The listing builds one solid part. Answer for the finished solid, in the listing's coordinates (mm). A direction names the side the tool comes from. Coordinates: 2 decimals unless noted, no trailing zeros. Order: outer loops, then holes, each group sorted by start corner. A loop starts at its lowest first (then second) coordinate and runs counter-clockwise, first axis right, second up. Notation, with made-up numbers: (56.25, -14) -> (83.25, -14) arc R25 ccw to (83.25, -2) -> close; hole circle Ø6 at (72.5, -29.75). An arc over 180 degrees is marked (long way). Write item = value, one per line.
from build123d import *

# Parameters (mm, degrees)
BOSS_EXTRU_1_DEPTH           = 2000
ENL_V_MAT_EXTRU_1_DEPTH      = 2000
ENL_V_MAT_EXTRU_2_DEPTH      = 2000
ENL_V_MAT_EXTRU_3_DEPTH      = 2000
ENL_V_MAT_EXTRU_4_DEPTH      = 2933
ENL_V_MAT_EXTRU_5_DEPTH      = 2933
ENL_V_MAT_EXTRU_5_DEPTH_BACK = 2933
ENL_V_MAT_EXTRU_6_DEPTH      = 50
ENL_V_MAT_EXTRU_7_DEPTH      = 1023
ENL_V_MAT_EXTRU_8_DEPTH      = 50
ESQUISSE14_W                 = 94.610765079
ESQUISSE14_H                 = 3.897152032
BOSS_EXTRU_2_DEPTH           = 5
BOSS_EXTRU_28_START          = -6
BOSS_EXTRU_28_DEPTH          = 26
ESQUISSE12_R                 = 5
BOSS_EXTRU_29_DEPTH          = 20


with BuildPart() as part:
    # Esquisse1 → Boss.-Extru.1 (new body)
    with BuildSketch(Plane(origin=(0, 0, 0), x_dir=(0, 0, -1), z_dir=(1, 0, 0))):
        Polygon((-880.445159684, -98.858699346), (-480.445159684, 601.141300654), (619.554840316, 901.141300654), (619.554840316, -598.858699346), (-880.445159684, -598.858699346), align=None)
    extrude(amount=BOSS_EXTRU_1_DEPTH)

    # Esquisse2 → Enlèv. mat.-Extru.1 (cut)
    with BuildSketch(Plane.XZ.offset(598.858699346)):
        Polygon((2000, -619.554840316), (1800, 880.445159684), (2000, 880.445159684), align=None)
        Polygon((200, 880.445159684), (0, 880.445159684), (0, -619.554840316), align=None)
    extrude(amount=-ENL_V_MAT_EXTRU_1_DEPTH, mode=Mode.SUBTRACT)

    # Esquisse4 → Enlèv. mat.-Extru.2 (cut)
    with BuildSketch(Plane(origin=(116.098887378, 0, -870.741655333), x_dir=(0, 1, 0), z_dir=(0.13216372009101793, 0, -0.9912279006826347))):
        Polygon((-598.858699346, 1900.573128869), (901.141300654, 1900.573128869), (901.141300654, 1800.573128869), align=None)
    extrude(amount=-ENL_V_MAT_EXTRU_2_DEPTH, mode=Mode.SUBTRACT)

    # Esquisse5 → Enlèv. mat.-Extru.3 (cut)
    with BuildSketch(Plane(origin=(-81.164389561, 0, -608.732921708), x_dir=(0, 1, 0), z_dir=(0.13216372009101793, 0, 0.9912279006826347))):
        Polygon((901.141300654, -81.882672497), (-598.858699346, -81.882672497), (901.141300654, -181.882672497), align=None)
    extrude(amount=ENL_V_MAT_EXTRU_3_DEPTH, mode=Mode.SUBTRACT)

    # Esquisse6 → Enlèv. mat.-Extru.4 (cut)
    with BuildSketch(Plane(origin=(0, 0, 0), x_dir=(0, 0, -1), z_dir=(1, 0, 0))):
        Polygon((569.554840316, 835.678781331), (-447.308376432, 558.35244949), (-830.445159684, -112.1369212), (-830.445159684, -548.858699346), (569.554840316, -548.858699346), align=None)
    extrude(amount=ENL_V_MAT_EXTRU_4_DEPTH, mode=Mode.SUBTRACT)

    # Esquisse7 → Enlèv. mat.-Extru.5 (cut, two sides: drawn at the far end of the back side and taken through both)
    with BuildSketch(Plane.XY.offset(-ENL_V_MAT_EXTRU_5_DEPTH_BACK)):
        Polygon((282.05986694, -123.858699346), (253.475791256, -548.858699346), (1746.524208744, -548.858699346), (1717.94013306, -123.858699346), align=None)
        Polygon((283.406973938, -73.858699346), (1716.593026062, -73.858699346), (1722.400013951, 576.141300654), (277.599986049, 576.141300654), align=None)
        Polygon((176.229227458, 851.141300654), (271.096481507, 626.141300654), (1728.903518493, 626.141300654), (1823.770772542, 851.141300654), align=None)
    extrude(amount=ENL_V_MAT_EXTRU_5_DEPTH + ENL_V_MAT_EXTRU_5_DEPTH_BACK, mode=Mode.SUBTRACT)

    # Esquisse8 → Enlèv. mat.-Extru.6 (cut)
    with BuildSketch(Plane(origin=(0, 0, -619.554840316), x_dir=(-1, 0, 0), z_dir=(0, 0, -1))):
        Polygon((-1852.364900608, 851.141300654), (-1946.524208744, -548.858699346), (-53.475791256, -548.858699346), (-147.635099392, 851.141300654), align=None)
    extrude(amount=-ENL_V_MAT_EXTRU_6_DEPTH, mode=Mode.SUBTRACT)

    # Esquisse9 → Enlèv. mat.-Extru.7 (cut)
    with BuildSketch(Plane(origin=(0, 0, 0), x_dir=(1, 0, 0), z_dir=(0, 1, 0))):
        Polygon((156.96398896, 569.554840316), (271.954599929, -430.445159684), (1728.045400071, -430.445159684), (1843.03601104, 569.554840316), align=None)
    extrude(amount=ENL_V_MAT_EXTRU_7_DEPTH, mode=Mode.SUBTRACT)

    # Esquisse10 → Enlèv. mat.-Extru.8 (cut)
    with BuildSketch(Plane.XZ.offset(598.858699346)):
        Polygon((243.775819835, 830.445159684), (57.109153168, -569.554840316), (1942.890846832, -569.554840316), (1756.224180165, 830.445159684), align=None)
    extrude(amount=-ENL_V_MAT_EXTRU_8_DEPTH, mode=Mode.SUBTRACT)

    # Esquisse14 → Boss.-Extru.2 (add)
    with BuildSketch(Plane(origin=(1834.339717588, 0, 244.578629012), x_dir=(-0.13216372009101796, 0, 0.9912279006826348), z_dir=(-0.9912279006826348, 0, -0.13216372009101796))):
        with Locations((543.745908762, -550.807275362)):
            Rectangle(ESQUISSE14_W, ESQUISSE14_H)
    boss_extru_2 = extrude(amount=BOSS_EXTRU_2_DEPTH)

    # Esquisse15 → Boss.-Extru.28 (add)
    with BuildSketch(Plane(origin=(0, -548.858699346, 0), x_dir=(1, 0, 0), z_dir=(0, 1, 0)).offset(BOSS_EXTRU_28_START)):
        Polygon((1768.728290839, -736.664329633), (1763.772151335, -736.003511032), (1751.203848273, -830.563782674), (1756.224180165, -831.231050773), align=None)
    boss_extru_28 = extrude(amount=BOSS_EXTRU_28_DEPTH)

    # Esquisse12 → Boss.-Extru.29 (add)
    with BuildSketch(Plane(origin=(0, -548.858699346, 0), x_dir=(1, 0, 0), z_dir=(0, 1, 0))):
        with Locations(Location((1965.090614868, 559.554840316, 0), (0, 0, 270))):
            Circle(ESQUISSE12_R)
    boss_extru_29 = extrude(amount=BOSS_EXTRU_29_DEPTH)

    # Symétrie1: Boss.-Extru.2, Boss.-Extru.28, Boss.-Extru.29 across plane
    add(boss_extru_2.mirror(Plane(origin=(1000, 0, 0), x_dir=(0, 0, 1), z_dir=(1, 0, 0))))
    add(boss_extru_28.mirror(Plane(origin=(1000, 0, 0), x_dir=(0, 0, 1), z_dir=(1, 0, 0))))
    add(boss_extru_29.mirror(Plane(origin=(1000, 0, 0), x_dir=(0, 0, 1), z_dir=(1, 0, 0))))


solid = part.part
Q1. Section B-B, the plane x = 569 is taken. Give the vertices of the cut face in (y, z).
The answers:
outline = (-598.86, -619.55) -> (-548.86, -619.55) -> (-548.86, -569.55) -> (-598.86, -569.55) -> close; (-598.86, 830.45) -> (-548.86, 830.45) -> (-548.86, 880.45) -> (-598.86, 880.45) -> close; (-123.86, 830.45) -> (-112.14, 830.45) -> (-73.86, 808.57) -> (-73.86, 866.16) -> (-98.86, 880.45) -> (-123.86, 880.45) -> close; (576.14, 430.45) -> (614.78, 430.45) -> (601.14, 480.45) -> (576.14, 494.73) -> close; (851.14, -619.55) -> (901.14, -619.55) -> (887.5, -569.55) -> (851.14, -569.55) -> close
Q2. Section A-A, the plane z = -178.5 is taken. Give the vertices of the cut face in (x, y).
The answers:
outline = (58.81, -598.86) -> (109.25, -598.86) -> (109.25, -548.86) -> (62.17, -548.86) -> close; (148.12, 729.03) -> (201.93, 729.03) -> (201.93, 780.85) -> (151.6, 780.85) -> close; (1798.07, 729.03) -> (1851.88, 729.03) -> (1848.4, 780.85) -> (1798.07, 780.85) -> close; (1890.75, -598.86) -> (1941.19, -598.86) -> (1937.83, -548.86) -> (1890.75, -548.86) -> close
Q3. Find the intervals of material crossed by line 1 along Z through (x, y) = (1721.5, 15), in increasing order.
The answers:
line_1 = 757.8 to 815.38
Q4. Section C-C, the plane y = 707 is taken. Give the vertices of the cut face in (x, z), plus the area to 3 significant figures.
The answers:
outline = (87.83, -619.55) -> (137.94, -619.55) -> (137.94, -569.55) -> (94.49, -569.55) -> close; (157.4, -97.73) -> (211.22, -97.73) -> (233.07, 92.3) -> (182.74, 92.3) -> close; (1766.93, 92.3) -> (1788.78, -97.73) -> (1842.6, -97.73) -> (1817.26, 92.3) -> close; (1862.06, -619.55) -> (1912.17, -619.55) -> (1905.51, -569.55) -> (1862.06, -569.55) -> close
area = 24,500 mm2
Q5. A tool of negligible diameter and unlimited length cuts with its end or side. For faces 1 (the face through (1809.139, 697.663, -63.496)), 2 (the face through (996, -553, 830.445)), 3 (the face through (267.97, -333.38, 855.1)), 4 (the face through (995.804, 894.886, -596.618)), from which of +Z, -Z, +X, -X, +Y, -Y can it reach the whole face along a straight path? Write none if from no direction.
The answers:
face_1 = +X, -X, -Y
face_2 = none
face_3 = +Z, -Z
face_4 = +Z, +X, -X, +Y
Q6. Each of these flat-tipped pins is pushed along its axis until it touches: pin 1 Ø11.5 at (x, y) = (1848, 841) entering from -Z; pin 2 Ø5 at (x, y) = (905.5, -97) entering from -Z; pin 3 Ø9 at (x, z) = (1757.5, 782.5) entering from +Y; pin 4 Ø9 at (x, z) = (244, 775) entering from +Y. Where does it stop, or does it pass through?
The answers:
pin_1 = -619.55
pin_2 = 820.37
pin_3 = 80.42
pin_4 = 93.55
Q7. The mould has two halves that part along Y. Classify faces 5 (the face through (214.19, 736.49, -71.89)), 6 (the face through (99.896, 141.341, -594.905)), 7 (the face through (848, -548.859, -574)), 8 (the face through (1069, -598.859, -595)): released by +Y, released by -Y, zero draft, split by the parting line, or undercut.
The answers:
face_5 = zero draft
face_6 = undercut
face_7 = undercut
face_8 = released by -Y
